CAD build for the part. Positions are in the model's coordinates, mm. A direction names the side the tool comes from. Coordinates: 2 decimals unless noted, no trailing zeros. Write each loop counter-clockwise with the first axis right and the second up, starting at its lowest first coordinate (ties: lowest second). Pieces come first, ordered by that corner, then holes. Notation, with made-up numbers: (-19, 28) -> (23, 28) arc R15 cw to (23, 47) -> close; hole circle Ø3 at (78, 20.5). An arc over 180 degrees is marked (long way). Answer as CSV lines item,"result".
Autodesk Inventor part; units mm, degrees
ref_plane "YZ Plane" through (0, 0, 0) normal (1, 0, 0) x (0, 1, 0)
ref_plane "XZ Plane" through (0, 0, 0) normal (0, 1, 0) x (-1, 0, 0)
ref_plane "XY Plane" through (0, 0, 0) normal (0, 0, 1) x (1, 0, 0)
sketch "Sketch2" plane through (0, 0, 0) normal (0, 1, 0) x (-1, 0, 0)
  arc A0 (21.75, 12.5) -> (28.25, 12.5) centre (25, 12.5) ccw
  line L0 (28.25, 12.5) -> (21.75, 12.5) construction
  line L1 (28.25, 12.5) -> (34.75, 12.5) construction
  line L2 (28.25, 12.5) -> (28.25, 25)
  line L3 (28.25, 12.5) -> (40.75, 12.5) construction
  line L4 (21.75, 12.5) -> (21.75, 25)
  line L5 (21.75, 12.5) -> (34.25, 12.5) construction
  arc A1 (28.25, 25) -> (21.75, 25) centre (25, 25) ccw
  arc A2 (-53.25, 12.5) -> (-46.75, 12.5) centre (-50, 12.5) ccw
  line L6 (-46.75, 12.5) -> (-53.25, 12.5) construction
  line L7 (-46.75, 12.5) -> (-40.25, 12.5) construction
  line L8 (-46.75, 12.5) -> (-46.75, 25)
  line L9 (-46.75, 12.5) -> (-34.25, 12.5) construction
  line L10 (-53.25, 12.5) -> (-53.25, 25)
  line L11 (-53.25, 12.5) -> (-40.75, 12.5) construction
  arc A3 (-46.75, 25) -> (-53.25, 25) centre (-50, 25) ccw
  arc A4 (-53.25, -62.5) -> (-46.75, -62.5) centre (-50, -62.5) ccw
  line L12 (-46.75, -62.5) -> (-53.25, -62.5) construction
  line L13 (-46.75, -62.5) -> (-40.25, -62.5) construction
  line L14 (-46.75, -62.5) -> (-46.75, -50)
  line L15 (-46.75, -62.5) -> (-34.25, -62.5) construction
  line L16 (-53.25, -62.5) -> (-53.25, -50)
  line L17 (-53.25, -62.5) -> (-40.75, -62.5) construction
  arc A5 (-46.75, -50) -> (-53.25, -50) centre (-50, -50) ccw
  line L18 (28.25, -62.5) -> (40.75, -62.5) construction
  line L19 (28.25, -62.5) -> (34.75, -62.5) construction
  line L20 (28.25, -62.5) -> (28.25, -50)
  line L21 (21.75, -62.5) -> (34.25, -62.5) construction
  arc A6 (21.75, -62.5) -> (28.25, -62.5) centre (25, -62.5) ccw
  line L22 (28.25, -62.5) -> (21.75, -62.5) construction
  line L23 (21.75, -62.5) -> (21.75, -50)
  arc A7 (28.25, -50) -> (21.75, -50) centre (25, -50) ccw
  line L24 (33, 33) -> (-58, 33)
  line L25 (-58, 33) -> (-58, -70.5)
  line L26 (-58, -70.5) -> (33, -70.5)
  line L27 (33, -70.5) -> (33, 33)
  circle A8 centre (-12.5, -33.75) radius 3
  point P0 (0, 0)
  dimension "d25" = 6.5
  dimension "d26" = 180
  dimension "d27" = 3.25
  dimension "d28" = 12.5
  dimension "d29" = 90
  dimension "d30" = 12.5
  dimension "d31" = 90
  dimension "d32" = 3.25
  dimension "d33" = 6.5
  dimension "d34" = 180
  dimension "d35" = 3.25
  dimension "d36" = 12.5
  dimension "d37" = 90
  dimension "d38" = 12.5
  dimension "d39" = 90
  dimension "d40" = 3.25
  dimension "d41" = 25
  dimension "d42" = 25
  dimension "d43" = 6.5
  dimension "d44" = 180
  dimension "d45" = 3.25
  dimension "d46" = 12.5
  dimension "d47" = 90
  dimension "d48" = 12.5
  dimension "d49" = 90
  dimension "d50" = 3.25
  dimension "d51" = 6.5
  dimension "d52" = 180
  dimension "d53" = 3.25
  dimension "d54" = 12.5
  dimension "d55" = 90
  dimension "d56" = 12.5
  dimension "d57" = 90
  dimension "d58" = 3.25
  dimension "d59" = 75
  dimension "d60" = 0
  dimension "d61" = 75
  dimension "d62" = 0
  dimension "d63" = 75
  dimension "d64" = 75
  dimension "d65" = 8
  dimension "d66" = 8
  dimension "d67" = 8
  dimension "d68" = 8
  dimension "d71" = 6
  dimension "d76" = 16.25
  dimension "d77" = 37.5
extrude "Extrusion2" add sketch "Sketch2" along normal blind 10
properties part number "StepperAdapter"
Item 1: Two-plate mould, pull along X, no slides. Class faces 1 (the flat face through (58, 5, -18)), 2 (the flat face through (-21.75, 5, 19)), 3 (the flat face through (-33, 5, -19)): pulls with the +X half, pulls with the -X half, needs draft (parallel to the pull), parting line crosses it, or undercut.
Answer below:
face 1,"pulls with the +X half"
face 2,"undercut"
face 3,"pulls with the -X half"
Item 2: Saw through at D-D on x = 12.5. Give the cut face in (y, z).
Answer below:
outline,"(0, -70.5) -> (10, -70.5) -> (10, -36.75) -> (0, -36.75) -> close; (0, -30.75) -> (10, -30.75) -> (10, 33) -> (0, 33) -> close"
Item 3: Flat gauge pins, fed straight in: pin 1 (5 mm diameter, centred on x = 39, z = -37.5, fed in from -Y); pin 2 (5 mm diameter, centred on x = 12.5, z = -33.75, fed in from -Y). Where does each tip first touch, or does it go through?
Answer below:
pin 1,"stops at y = 0"
pin 2,"passes through"
Item 4: Saw through at C-C on y = 1.5. Give the cut face in (x, z), and give its area (3 significant figures).
Answer below:
outline,"(-33, -70.5) -> (58, -70.5) -> (58, 33) -> (-33, 33) -> close; hole (-28.25, -62.5) arc R3.25 ccw to (-21.75, -62.5) -> (-21.75, -50) arc R3.25 ccw to (-28.25, -50) -> close; hole (-28.25, 12.5) arc R3.25 ccw to (-21.75, 12.5) -> (-21.75, 25) arc R3.25 ccw to (-28.25, 25) -> close; hole circle Ø6 at (12.5, -33.75); hole (46.75, -62.5) arc R3.25 ccw to (53.25, -62.5) -> (53.25, -50) arc R3.25 ccw to (46.75, -50) -> close; hole (46.75, 12.5) arc R3.25 ccw to (53.25, 12.5) -> (53.25, 25) arc R3.25 ccw to (46.75, 25) -> close"
area,"8,930 mm2"
Item 5: 3-axis set-ups, long thin cutter, end or side, ignore diameter. For faces 4 (the flat face through (13, 5, -70.5)), 5 (the flat face through (46.75, 5, 19)): which of +Z, -Z, +X, -X, +Y, -Y reach the whole face in a straight line?
Answer below:
face 4,"-Z, +X, -X, +Y, -Y"
face 5,"+Y, -Y"
Item 6: Saw through at A-A on x = -25. Give the cut face in (y, z), and give its area (3 significant figures).
Answer below:
outline,"(0, -70.5) -> (10, -70.5) -> (10, -65.75) -> (0, -65.75) -> close; (0, -46.75) -> (10, -46.75) -> (10, 9.25) -> (0, 9.25) -> close; (0, 28.25) -> (10, 28.25) -> (10, 33) -> (0, 33) -> close"
area,"655 mm2"
Item 7: Wall check: line 1 (X direction, y = 7.5, z = 16.5); line 2 (Z direction, x = 12.5, y = 2.5); line 3 (Z direction, x = 50.5, y = 5.5). Give the ranges that are in metal, low to high. Write a range as from..to.
Answer below:
line 1,"x = -33..-28.25, -21.75..46.75, 53.25..58"
line 2,"z = -70.5..-36.75, -30.75..33"
line 3,"z = -70.5..-65.71, -46.79..9.29, 28.21..33"
Item 8: Saw through at B-B on z = -33.75. Give the cut face in (x, y), and give its area (3 significant figures).
Answer below:
outline,"(-33, 0) -> (9.5, 0) -> (9.5, 10) -> (-33, 10) -> close; (15.5, 0) -> (58, 0) -> (58, 10) -> (15.5, 10) -> close"
area,"850 mm2"
